The listing builds one solid part. Answer for the finished solid, in the listing's coordinates (mm). Face numbers are marked on the shaded views. A direction names the side the tool comes from. Coordinates: 2 decimals unless noted, no trailing zeros. Order: outer loops, then holes, each group sorted by start corner. A loop starts at its lowest first (then second) coordinate and runs counter-clockwise, first axis right, second up.
```python
from build123d import *

# Parameters (mm, degrees)
SKETCH1_W           = 20
SKETCH1_H           = 40
BOSS_EXTRUDE1_DEPTH = 80
SKETCH8_W           = 25
SKETCH8_H           = 64
BOSS_EXTRUDE2_DEPTH = 57
SKETCH12_W          = 57
SKETCH12_H          = 6
BOSS_EXTRUDE3_DEPTH = 8
SKETCH14_W          = 57
SKETCH14_H          = 6
BOSS_EXTRUDE4_DEPTH = 8
SKETCH17_W          = 48
SKETCH17_H          = 80
CUT_EXTRUDE4_DEPTH  = 36
CHAMFER1_SIZE       = 10
SKETCH16_W          = 48
SKETCH16_H          = 72
CUT_EXTRUDE5_DEPTH  = 10
SKETCH19_R          = 1.25
CUT_EXTRUDE6_DEPTH  = 109.102562738
SKETCH21_W          = 19
SKETCH21_H          = 53
CUT_EXTRUDE7_DEPTH  = 108.916413596
SKETCH22_R          = 4.25
CUT_EXTRUDE8_DEPTH  = 103.323819663
SKETCH25_W          = 3
SKETCH25_H          = 8
SKETCH25_H_2        = 53
CUT_EXTRUDE11_DEPTH = 108.916413596


with BuildPart() as part:
    # Sketch1 → Boss-Extrude1 (new body)
    with BuildSketch(Plane(origin=(0, 0, 0), x_dir=(1, 0, 0), z_dir=(0, 1, 0))):
        Polygon((-17.351649908, 20.312727502), (-57.351649908, -19.687272498), (-17.351649908, -19.687272498), align=None)
        with Locations((-7.351649908, 0.312727502)):
            Rectangle(SKETCH1_W, SKETCH1_H)
    extrude(amount=-BOSS_EXTRUDE1_DEPTH)

    # Sketch8 → Boss-Extrude2 (add)
    with BuildSketch(Plane(origin=(2.648350092, 0, 0), x_dir=(0, 0, -1), z_dir=(1, 0, 0))):
        with Locations((-32.187272498, -40)):
            Rectangle(SKETCH8_W, SKETCH8_H)
    extrude(amount=-BOSS_EXTRUDE2_DEPTH)

    # Sketch12 → Boss-Extrude3 (add)
    with BuildSketch(Plane.XZ.offset(72)):
        with Locations((-25.851649908, 41.687272498)):
            Rectangle(SKETCH12_W, SKETCH12_H)
    extrude(amount=BOSS_EXTRUDE3_DEPTH)

    # Sketch14 → Boss-Extrude4 (add)
    with BuildSketch(Plane(origin=(0, -8, 0), x_dir=(1, 0, 0), z_dir=(0, 1, 0))):
        with Locations((-25.851649908, -41.687272498)):
            Rectangle(SKETCH14_W, SKETCH14_H)
    extrude(amount=BOSS_EXTRUDE4_DEPTH)

    # Sketch17 → Cut-Extrude4 (cut)
    with BuildSketch(Plane(origin=(0, 0, -20.312727502), x_dir=(-1, 0, 0), z_dir=(0, 0, -1))):
        with Locations((29.351649908, -40)):
            Rectangle(SKETCH17_W, SKETCH17_H)
    extrude(amount=-CUT_EXTRUDE4_DEPTH, mode=Mode.SUBTRACT)

    # Chamfer1
    chamfer1_edges = [part.edges().sort_by_distance(p)[0] for p in [
        (-5.351649908, -40, 15.687272498),
    ]]
    chamfer(chamfer1_edges, length=CHAMFER1_SIZE)

    # Sketch16 → Cut-Extrude5 (cut)
    with BuildSketch(Plane(origin=(0, 0, 15.687272498), x_dir=(-1, 0, 0), z_dir=(0, 0, -1))):
        with Locations((29.351649908, -40)):
            Rectangle(SKETCH16_W, SKETCH16_H)
    extrude(amount=CUT_EXTRUDE5_DEPTH, mode=Mode.SUBTRACT)

    # Sketch19 → Cut-Extrude6 (cut, through all)
    with BuildSketch(Plane(origin=(0, 0, 0), x_dir=(1, 0, 0), z_dir=(0, 1, 0))):
        with Locations(Location((-7.851649908, -13.187272498, 0), (0, 0, 270))):
            Circle(SKETCH19_R)
    extrude(amount=-CUT_EXTRUDE6_DEPTH, mode=Mode.SUBTRACT)

    # Sketch21 → Cut-Extrude7 (cut, through all)
    with BuildSketch(Plane.ZY.offset(54.351649908)):
        with Locations((29.187272498, -40)):
            Rectangle(SKETCH21_W, SKETCH21_H)
    extrude(amount=-CUT_EXTRUDE7_DEPTH, mode=Mode.SUBTRACT)

    # Sketch22 → Cut-Extrude8 (cut, through all)
    with BuildSketch(Plane.XZ.offset(72)):
        with Locations(Location((-45.351649908, 29.187272498, 0), (0, 0, 270))):
            Circle(SKETCH22_R)
    extrude(amount=-CUT_EXTRUDE8_DEPTH, mode=Mode.SUBTRACT)

    # Sketch25 → Cut-Extrude11 (cut, through all)
    with BuildSketch(Plane.ZY.offset(54.351649908)):
        with Locations((40.187272498, -76)):
            Rectangle(SKETCH25_W, SKETCH25_H)
        with Locations((40.187272498, -40)):
            Rectangle(SKETCH25_W, SKETCH25_H_2)
        with Locations((40.187272498, -4)):
            Rectangle(SKETCH25_W, SKETCH25_H)
    extrude(amount=-CUT_EXTRUDE11_DEPTH, mode=Mode.SUBTRACT)


solid = part.part
```
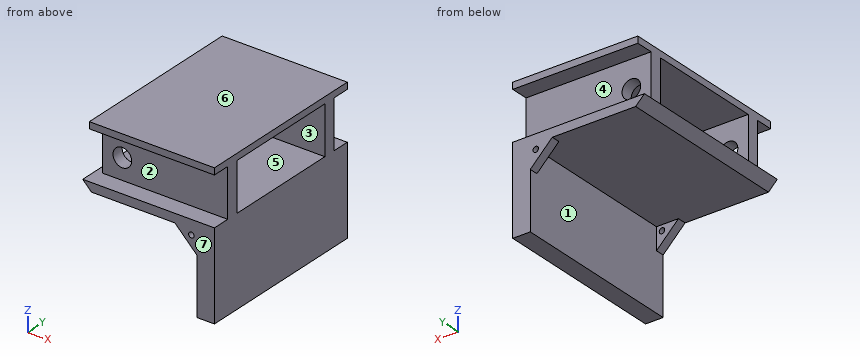
(1) Consider line 1 (Z direction, x = -29, y = -59); line 2 (Y direction, x = -45.5, z = 40); line 3 (X direction, y = -37.5, z = 5). Determine where each line is inside the solid, lowest interval first.
(2) The mould has two halves that part along Z. Classify the marked faces 5, 6 and 7: released by +Z, released by -Z, zero draft, split by the parting line, or undercut.
(3) Find section A-A (z = 30). Write down the section's boundary in (x, y).
(4) Find section D-D (y = -69). Write down the section's boundary in (x, z).
(5) Find section B-B (y = -31). Write down the section's boundary in (x, z).
(6) For the marked faces 1, 2, 3 and 4, determine the directions among +Z, -Z, +X, -X, +Y, -Y from which every point of the face is accessible in a straight line to the end or side of a thin tool.
(7) Find section C-C (x = -35). Write down the section's boundary in (y, z), and give its area (3 significant figures).
(8) Each of these flat-tipped pins is pushed along its axis until it touches: pin 1 Ø11 at (x, z) = (-45.35, 29.19) entering from -Y; pin 2 Ø6.5 at (x, y) = (-29, -4.5) entering from -Z; pin 3 Ø6.5 at (x, z) = (-17, 35) entering from +Y. Where does it stop, or does it pass through?
Findings below:
1. line 1: z = 15.69 to 19.69, 41.69 to 44.69
1. line 2: y = -72 to -66.5, -13.5 to -8
1. line 3: x = -5.35 to 2.65
2. face 5: undercut
2. face 6: released by +Z
2. face 7: zero draft
3. outline: (-54.35, -72) - (-49.52, -72) - (-49.52, -66.5) - (-54.35, -66.5) - close; (-54.35, -13.5) - (-49.52, -13.5) - (-49.52, -8) - (-54.35, -8) - close; (-41.18, -72) - (2.65, -72) - (2.65, -66.5) - (-41.18, -66.5) - close; (-41.18, -13.5) - (2.65, -13.5) - (2.65, -8) - (-41.18, -8) - close
4. outline: (-57.35, 19.69) - (-53.35, 15.69) - (-5.35, 15.69) - (-5.35, -20.31) - (2.65, -20.31) - (2.65, 44.69) - (-54.35, 44.69) - (-54.35, 19.69) - close; hole circle Ø8.5 at (-45.35, 29.19)
5. outline: (-57.35, 19.69) - (-53.35, 15.69) - (-5.35, 15.69) - (-5.35, -20.31) - (2.65, -20.31) - (2.65, 19.69) - close; (-54.35, 41.69) - (2.65, 41.69) - (2.65, 44.69) - (-54.35, 44.69) - close
6. face 1: -Z, -X
6. face 2: +X, -X, -Y
6. face 3: +X, -X
6. face 4: +X, -X, +Y
7. outline: (-80, 15.69) - (0, 15.69) - (0, 19.69) - (-8, 19.69) - (-8, 41.69) - (0, 41.69) - (0, 44.69) - (-80, 44.69) - (-80, 41.69) - (-72, 41.69) - (-72, 19.69) - (-80, 19.69) - close; hole (-66.5, 19.69) - (-13.5, 19.69) - (-13.5, 41.69) - (-66.5, 41.69) - close
7. area: 802 mm2
8. pin 1: stops at y = -72
8. pin 2: stops at z = 15.69
8. pin 3: stops at y = -8
